Read the model definition and answer for the solid it produces. Units are mm, in the model's axes. A direction names the side the tool comes from. Coordinates: 2 decimals unless noted, no trailing zeros. Write each loop counter-clockwise with the first axis right and the second up, starting at its lowest first coordinate (ties: lowest second). Pieces come first, ordered by that corner, then holes.
(1) Which of the six approach directions +Z, -Z, +X, -X, +Y, -Y give full straight-line access (tool end or side, diameter ignored) to faces 1 (the cylindrical face through (40.2, 5.1, 15.5)), 2 (the flat face through (62.204, -27.619, 9.154)), 3 (the flat face through (-18.279, 18.617, 9.86)), 4 (the cylindrical face through (59.5, -32.6, 10.1)), 5 (the flat face through (23.87, 12.8, -0.99))?
(2) The part is cut by section A-A, the plane y = 0. Determine the outline of the cut face in (x, z), and give its area (3 significant figures).
(3) Straight lines are drawn through the part: line 1 along Z through (x, y) = (71.25, -63); line 2 along Y through (x, z) = (6, 12.25); line 3 along X through (y, z) = (-13.5, 9.5). For each, find the intervals that lie inside material, in ascending order.
(4) Determine the mould class of faces 6 (the flat face through (-59.447, -26.408, 7.638)), 7 (the cylindrical face through (-46.8, -76.53, 8.05)) for opening direction Y: pulls with the +Y half, pulls with the -Y half, needs draft (parallel to the pull), parting line crosses it, or undercut.
(5) Given pin 1 (3 mm diameter, centred on y = -30.5, z = 6.5, fed in from -X); pin 2 (2 mm diameter, centred on x = 36, z = -1, fed in from +Y); pin 3 (10 mm diameter, centred on x = -4.5, y = 14, fed in from +Z), each flat-ended and moving along its own axis, determine where each tip first touches the part or whether it passes through.
(6) The part is cut by section D-D, the plane x = -26. Determine the outline of the cut face in (y, z), and give its area (3 significant figures).
(7) The part is cut by section B-B, the plane x = 8. Determine the outline of the cut face in (y, z), and give its area (3 significant figures).
(8) The part is cut by section C-C, the plane y = -63. Determine the outline of the cut face in (x, z).
```python
from build123d import *

# Parameters (mm, degrees)
EXTRUDE_THIN3_DEPTH     = 20
SKETCH5_W               = 20.5
SKETCH5_H               = 20.5
BOSS_EXTRUDE2_DEPTH     = 2
SKETCH6_R               = 5.1
CUT_EXTRUDE1_DEPTH      = 5
CUT_EXTRUDE2_DEPTH      = 113.143625411
CUT_EXTRUDE2_DEPTH_BACK = 113.143625411
SKETCH7_R               = 7.5
SKETCH7_R_2             = 6.5
CUT_EXTRUDE3_DEPTH      = 113.143625411
CUT_EXTRUDE3_DEPTH_BACK = 113.143625411
SKETCH8_R               = 7.5
SKETCH9_R               = 7.5
CUT_EXTRUDE4_DEPTH      = 5
SKETCH10_R              = 7.5
CUT_EXTRUDE5_DEPTH      = 5


with BuildPart() as part:
    # Sketch4 → Extrude-Thin3 (new body)
    with BuildSketch(Plane.XY):
        Polygon((68.26921232, -78.007734737), (-68.26921232, -78.007734737), (-78.04476947, -49.332767098), (-59.641599788, -35.135114275), (-64.69543331, -20.310535944), (-41.7225, -15.181760387), (-41.7225, 13.794543937), (-10.635850775, 24.392265263), (10.635850775, 24.392265263), (41.7225, 13.794543937), (41.7225, -15.181760387), (64.69543331, -20.310535944), (59.641599788, -35.135114275), (78.04476947, -49.332767098), align=None)
        Polygon((66.122401602, -75.007734737), (-66.122401602, -75.007734737), (-74.512519059, -50.396723531), (-56.109349377, -36.199070708), (-60.776273805, -22.509425719), (-38.7225, -17.58585525), (-38.7225, 11.647733219), (-10.138539336, 21.392265263), (10.138539336, 21.392265263), (38.7225, 11.647733219), (38.7225, -17.58585525), (60.776273805, -22.509425719), (56.109349377, -36.199070708), (74.512519059, -50.396723531), align=None, mode=Mode.SUBTRACT)
    extrude(amount=EXTRUDE_THIN3_DEPTH)

    # Sketch5 → Boss-Extrude2 (add)
    with BuildSketch(Plane.XY):
        Polygon((10.635850775, 24.392265263), (41.7225, 13.794543937), (41.7225, -15.181760387), (64.69543331, -20.310535944), (59.641599788, -35.135114275), (78.04476947, -49.332767098), (68.26921232, -78.007734737), (-68.26921232, -78.007734737), (-78.04476947, -49.332767098), (-59.641599788, -35.135114275), (-64.69543331, -20.310535944), (-41.7225, -15.181760387), (-41.7225, 13.794543937), (-10.635850775, 24.392265263), align=None)
        Rectangle(SKETCH5_W, SKETCH5_H, mode=Mode.SUBTRACT)
        Polygon((55.669537991, -26.0225), (48.169537991, -48.0225), (23.169537991, -48.0225), (15.669537991, -26.0225), align=None, mode=Mode.SUBTRACT)
        Polygon((-20, -48.0225), (20, -48.0225), (12.5, -26.0225), (-12.5, -26.0225), align=None, mode=Mode.SUBTRACT)
        Polygon((-15.669537991, -26.0225), (-23.169537991, -48.0225), (-48.169537991, -48.0225), (-55.669537991, -26.0225), align=None, mode=Mode.SUBTRACT)
        Polygon((13.0225, 16.5), (35.0225, 9), (35.0225, -16), (13.0225, -23.5), align=None, mode=Mode.SUBTRACT)
        Polygon((-35.0225, -16), (-13.0225, -23.5), (-13.0225, 16.5), (-35.0225, 9), align=None, mode=Mode.SUBTRACT)
        Polygon((-54.081215036, -39.978892106), (-69.782858952, -52.092375431), (-63.008353643, -71.964257668), (63.008353643, -71.964257668), (69.782858952, -52.092375431), (54.081215036, -39.978892106), (50.316348709, -51.0225), (-50.316348709, -51.0225), align=None, mode=Mode.SUBTRACT)
    extrude(amount=-BOSS_EXTRUDE2_DEPTH)

    # Sketch6 → Cut-Extrude1 (cut)
    with BuildSketch(Plane(origin=(0, 24.392265263, 0), x_dir=(1, 0, 0), z_dir=(0, 1, 0))):
        with Locations(Location((0, -10.000182073, 0), (0, 0, 180))):
            Circle(SKETCH6_R)
    extrude(amount=-CUT_EXTRUDE1_DEPTH, mode=Mode.SUBTRACT)

    # Sketch7 → Cut-Extrude2 (cut, two sides: drawn at the far end of the back side and taken through both)
    with BuildSketch(Plane(origin=(0, 0, 0), x_dir=(1, 0, 0), z_dir=(0, 1, 0)).offset(-CUT_EXTRUDE2_DEPTH_BACK)):
        with Locations((-26, -10)):
            Circle(SKETCH7_R)
        with Locations((-53, -10)):
            Circle(SKETCH7_R_2)
        with Locations(Location((26, -10, 0), (0, 0, 180))):
            Circle(SKETCH7_R)
        with Locations(Location((53, -10, 0), (0, 0, 180))):
            Circle(SKETCH7_R_2)
    extrude(amount=CUT_EXTRUDE2_DEPTH + CUT_EXTRUDE2_DEPTH_BACK, mode=Mode.SUBTRACT)

    # Sketch8 → Cut-Extrude3 (cut, two sides: drawn at the far end of the back side and taken through both)
    with BuildSketch(Plane(origin=(0, 0, 0), x_dir=(0, 0, -1), z_dir=(1, 0, 0)).offset(-CUT_EXTRUDE3_DEPTH_BACK)):
        with Locations((-10, 0)):
            Circle(SKETCH8_R)
        with Locations(Location((-10, -63, 0), (0, 0, 270))):
            Circle(SKETCH8_R)
    extrude(amount=CUT_EXTRUDE3_DEPTH + CUT_EXTRUDE3_DEPTH_BACK, mode=Mode.SUBTRACT)

    # Sketch9 → Cut-Extrude4 (cut)
    with BuildSketch(Plane(origin=(5.260509798, 6.818736564, 0), x_dir=(0.7917630726515511, -0.6108283202221183, 0), z_dir=(0.6108283202221182, 0.791763072651551, 0))):
        with Locations(Location((80, -10, 0), (0, 0, 180))):
            Circle(SKETCH9_R)
    extrude(amount=-CUT_EXTRUDE4_DEPTH, mode=Mode.SUBTRACT)

    # Sketch10 → Cut-Extrude5 (cut)
    with BuildSketch(Plane(origin=(-5.260509798, 6.818736564, 0), x_dir=(0.7917630726515507, 0.6108283202221189, 0), z_dir=(-0.6108283202221189, 0.7917630726515507, 0))):
        with Locations(Location((-80, -10, 0), (0, 0, 180))):
            Circle(SKETCH10_R)
    extrude(amount=-CUT_EXTRUDE5_DEPTH, mode=Mode.SUBTRACT)


solid = part.part
```
Computed:
1. face 1: +X, -X
1. face 2: +Z, -Z, +X
1. face 3: +Z
1. face 4: +Y, -Y
1. face 5: +Z, -Z
2. outline: (-41.72, -2) - (-35.02, -2) - (-35.02, 0) - (-38.72, 0) - (-38.72, 2.5) - (-41.72, 2.5) - close; (-41.72, 17.5) - (-38.72, 17.5) - (-38.72, 20) - (-41.72, 20) - close; (-13.02, -2) - (-10.25, -2) - (-10.25, 0) - (-13.02, 0) - close; (10.25, -2) - (13.02, -2) - (13.02, 0) - (10.25, 0) - close; (35.02, -2) - (41.72, -2) - (41.72, 2.5) - (38.72, 2.5) - (38.72, 0) - (35.02, 0) - close; (38.72, 17.5) - (41.72, 17.5) - (41.72, 20) - (38.72, 20) - close
2. area: 67.9 mm2
3. line 1: z = -2 to 2.5, 17.5 to 20
3. line 2: y = -78.01 to -75.01, 21.39 to 24.39
3. line 3: x = -41.72 to -38.72, 38.72 to 41.72
4. face 6: undercut
4. face 7: needs draft
5. pin 1: stops at x = -61.73
5. pin 2: stops at y = 16.09
5. pin 3: stops at z = 0
6. outline: (-78.01, -2) - (-71.96, -2) - (-71.96, 0) - (-75.01, 0) - (-75.01, 2.5) - (-78.01, 2.5) - close; (-78.01, 17.5) - (-75.01, 17.5) - (-75.01, 20) - (-78.01, 20) - close; (-51.02, -2) - (-48.02, -2) - (-48.02, 0) - (-51.02, 0) - close; (-26.02, -2) - (-19.08, -2) - (-19.08, 0) - (-26.02, 0) - close; (12.08, -2) - (19.15, -2) - (19.15, 2.5) - (15.98, 2.5) - (15.98, 0) - (12.08, 0) - close; (15.98, 17.5) - (19.15, 17.5) - (19.15, 20) - (15.98, 20) - close
6. area: 77.0 mm2
7. outline: (-78.01, -2) - (-71.96, -2) - (-71.96, 0) - (-75.01, 0) - (-75.01, 20) - (-78.01, 20) - close; (-51.02, -2) - (-48.02, -2) - (-48.02, 0) - (-51.02, 0) - close; (-26.02, -2) - (-10.25, -2) - (-10.25, 0) - (-26.02, 0) - close; (10.25, -2) - (24.39, -2) - (24.39, 20) - (21.39, 20) - (21.39, 0) - (10.25, 0) - close
7. area: 198 mm2
8. outline: (-73.39, -2) - (-66.06, -2) - (-66.06, 0) - (-70.22, 0) - (-70.22, 2.5) - (-73.39, 2.5) - close; (-73.39, 17.5) - (-70.22, 17.5) - (-70.22, 20) - (-73.39, 20) - close; (66.06, -2) - (73.39, -2) - (73.39, 2.5) - (70.22, 2.5) - (70.22, 0) - (66.06, 0) - close; (70.22, 17.5) - (73.39, 17.5) - (73.39, 20) - (70.22, 20) - close
